from build123d import *

# Parameters (mm, degrees)
SKETCH_1_W                 = 44
SKETCH_1_H                 = 78
EXTRUDE_1_DEPTH            = 35
SHELL_1_T                  = -3
SHELL_1_THICKNESS_2_FACE_W = 75
SHELL_1_THICKNESS_2_FACE_H = 38
SHELL_1_THICKNESS_2_DEPTH  = 7
SKETCH_3_R                 = 3.6
CUT_EXTRUDE_1_DEPTH        = 4.1
CUT_EXTRUDE_2_REACH        = 53.284
SKETCH_4_R                 = 2.25
SKETCH_5_W                 = 3
SKETCH_5_H                 = 3
CUT_EXTRUDE_3_DEPTH        = 6
SKETCH_6_W                 = 8
SKETCH_6_H                 = 8
SKETCH_6_R                 = 1.75
EXTRUDE_2_DEPTH            = 8
CUT_EXTRUDE_4_DEPTH        = 2.6
CUT_EXTRUDE_5_REACH        = 90.034
SKETCH_8_R                 = 5


with BuildPart() as part:
    # 草圖1 → 填料-伸長1 (new body)
    with BuildSketch(Plane(origin=(0, 0, 0), x_dir=(1, 0, 0), z_dir=(0, 1, 0))):
        Rectangle(SKETCH_1_W, SKETCH_1_H)
    extrude(amount=EXTRUDE_1_DEPTH)

    # 薄殼1
    shell_1_openings = [part.faces().sort_by_distance(p)[0] for p in [
        (0, 17.5, 39),
    ]]
    offset(amount=SHELL_1_T, openings=shell_1_openings, kind=Kind.INTERSECTION)

    # 薄殼1 thickness 2 face (on inner face of the shell) → 薄殼1 thickness 2 (add)
    with BuildSketch(Plane(origin=(0, 3, 1.5), x_dir=(0, 0, -1), z_dir=(0, -1, 0))):
        Rectangle(SHELL_1_THICKNESS_2_FACE_W, SHELL_1_THICKNESS_2_FACE_H)
    extrude(amount=-SHELL_1_THICKNESS_2_DEPTH)

    # 草圖3 → 除料-伸長1 (cut)
    with BuildSketch(Plane(origin=(0, 10, 0), x_dir=(1, 0, 0), z_dir=(0, 1, 0))):
        with Locations(Location((0, 25, 0), (0, 0, 270))):
            Circle(SKETCH_3_R)
        with Locations(Location((0, -29, 0), (0, 0, 270))):
            Circle(SKETCH_3_R)
    extrude(amount=-CUT_EXTRUDE_1_DEPTH, mode=Mode.SUBTRACT)

    # 草圖4 → 除料-伸長2 (cut, up to next)
    with BuildSketch(Plane(origin=(0, 10, 0), x_dir=(1, 0, 0), z_dir=(0, 1, 0)), mode=Mode.PRIVATE) as cut_extrude_2_sk1:
        with Locations(Location((0, 25, 0), (0, 0, 270))):
            Circle(SKETCH_4_R)
    cut_extrude_2_tool1 = extrude(cut_extrude_2_sk1.sketch, amount=-CUT_EXTRUDE_2_REACH, mode=Mode.PRIVATE) & part.part
    # 草圖4 → 除料-伸長2 (cut, up to next)
    with BuildSketch(Plane(origin=(0, 10, 0), x_dir=(1, 0, 0), z_dir=(0, 1, 0)), mode=Mode.PRIVATE) as cut_extrude_2_sk2:
        with Locations(Location((0, -29, 0), (0, 0, 270))):
            Circle(SKETCH_4_R)
    cut_extrude_2_tool2 = extrude(cut_extrude_2_sk2.sketch, amount=-CUT_EXTRUDE_2_REACH, mode=Mode.PRIVATE) & part.part
    add(cut_extrude_2_tool1.solids().sort_by_distance((0, 10, -25))[0], mode=Mode.SUBTRACT)
    add(cut_extrude_2_tool2.solids().sort_by_distance((0, 10, 29))[0], mode=Mode.SUBTRACT)

    # 草圖5 → 除料-伸長3 (cut)
    with BuildSketch(Plane.XY.offset(39)):
        with Locations((20.5, 11.5)):
            Rectangle(SKETCH_5_W, SKETCH_5_H)
    extrude(amount=-CUT_EXTRUDE_3_DEPTH, mode=Mode.SUBTRACT)

    # 草圖6 → 填料-伸長2 (add)
    with BuildSketch(Plane.XY.offset(39)):
        with Locations((-26, 31)):
            Rectangle(SKETCH_6_W, SKETCH_6_H)
        with Locations((-26, 31)):
            Circle(SKETCH_6_R, mode=Mode.SUBTRACT)
        with Locations((-26, 4)):
            Rectangle(SKETCH_6_W, SKETCH_6_H)
        with Locations((-26, 4)):
            Circle(SKETCH_6_R, mode=Mode.SUBTRACT)
        with Locations((26, 4)):
            Rectangle(SKETCH_6_W, SKETCH_6_H)
        with Locations(Location((26, 4, 0), (0, 0, 180))):
            Circle(SKETCH_6_R, mode=Mode.SUBTRACT)
        with Locations((26, 31)):
            Rectangle(SKETCH_6_W, SKETCH_6_H)
        with Locations(Location((26, 31, 0), (0, 0, 180))):
            Circle(SKETCH_6_R, mode=Mode.SUBTRACT)
    extrude(amount=-EXTRUDE_2_DEPTH)

    # 草圖7 → 除料-伸長4 (cut)
    with BuildSketch(Plane(origin=(0, 0, 31), x_dir=(-1, 0, 0), z_dir=(0, 0, -1))):
        Polygon((27.58771324, 6.75), (29.175426481, 4), (27.58771324, 1.25), (24.41228676, 1.25), (22.824573519, 4), (24.41228676, 6.75), align=None)
        Polygon((-22.824573519, 31), (-24.41228676, 33.75), (-27.58771324, 33.75), (-29.175426481, 31), (-27.58771324, 28.25), (-24.41228676, 28.25), align=None)
        Polygon((-29.175426481, 4), (-27.58771324, 1.25), (-24.41228676, 1.25), (-22.824573519, 4), (-24.41228676, 6.75), (-27.58771324, 6.75), align=None)
        Polygon((24.41228676, 28.25), (22.824573519, 31), (24.41228676, 33.75), (27.58771324, 33.75), (29.175426481, 31), (27.58771324, 28.25), align=None)
    extrude(amount=-CUT_EXTRUDE_4_DEPTH, mode=Mode.SUBTRACT)

    # 草圖8 → 除料-伸長5 (cut, up to next)
    with BuildSketch(Plane.XY.offset(-36), mode=Mode.PRIVATE) as cut_extrude_5_sk1:
        with Locations((0, 20)):
            Circle(SKETCH_8_R)
    cut_extrude_5_tool1 = extrude(cut_extrude_5_sk1.sketch, amount=-CUT_EXTRUDE_5_REACH, mode=Mode.PRIVATE) & part.part
    add(cut_extrude_5_tool1.solids().sort_by_distance((0, 20, -36))[0], mode=Mode.SUBTRACT)


solid = part.part
Geometry: final body of the model. Coordinates: model frame, mm. A direction names the side the tool comes from. Give positions to 0.01 mm unless a question says otherwise; leave off trailing zeros. Write each loop counter-clockwise with the first axis right and the second up, starting at its lowest first coordinate (ties: lowest second). Pieces come first, ordered by that corner, then holes. Notation, with made-up numbers: (89, 30) -> (132, 30) arc R17 cw to (132, 41) -> close; hole circle Ø1 at (-22.75, 30.5). An arc over 180 degrees is marked (long way). Answer in a Markdown table with one row per item.
(1) Pin query (flat end, axial travel): pin 1 (6.5 mm diameter, centred on x = -4, y = 26.5, fed in from +Z); pin 2 (6 mm diameter, centred on y = 9.5, z = 23.5, fed in from -X); pin 3 (3 mm diameter, centred on y = 14, z = 23, fed in from +X). Return the tip coordinate at first contact, or that it passes through.
Answers below:
| item | result |
|---|---|
| pin 1 | z = -36 |
| pin 2 | x = -22 |
| pin 3 | x = 22 |
(2) Section query A-A on x = 26. Return loops of the section in (y, z).
Answers below:
| item | result |
|---|---|
| outline | (0, 31) -> (1.25, 31) -> (1.25, 33.6) -> (2.25, 33.6) -> (2.25, 39) -> (0, 39) -> close; (5.75, 33.6) -> (6.75, 33.6) -> (6.75, 31) -> (8, 31) -> (8, 39) -> (5.75, 39) -> close; (27, 31) -> (28.25, 31) -> (28.25, 33.6) -> (29.25, 33.6) -> (29.25, 39) -> (27, 39) -> close; (32.75, 33.6) -> (33.75, 33.6) -> (33.75, 31) -> (35, 31) -> (35, 39) -> (32.75, 39) -> close |
(3) Ray query, line 1 along Y through (x, z) = (-11, -17.5); line 2 along X through (y, z) = (2, -25); line 3 along X through (y, z) = (22, -25). Return the intervals inside material, ascending. Write a range as [from, to].
Answers below:
| item | result |
|---|---|
| line 1 | [0, 10], [32, 35] |
| line 2 | [-22, -2.25], [2.25, 22] |
| line 3 | [-22, -19], [19, 22] |
(4) Section query D-D on z = 14. Return loops of the section in (x, y), then the cut area to 3 significant figures.
Answers below:
| item | result |
|---|---|
| outline | (-22, 0) -> (22, 0) -> (22, 35) -> (-22, 35) -> close; hole (-19, 10) -> (19, 10) -> (19, 32) -> (-19, 32) -> close |
| area | 704 mm^2 |
(5) Draft query along Y for faces 5 (the flat face through (-23.63, 29.606, 32.282)), 6 (the flat face through (0, 0, -1)), 7 (the flat face through (0, 13, -39)). Return one class per face: +Y half, -Y half, draft (parallel to the pull), parting line (faces both ways), or undercut.
Answers below:
| item | result |
|---|---|
| face 5 | undercut |
| face 6 | -Y half |
| face 7 | draft |
(6) Set-up query: faces 1 (the flat face through (23.63, 2.606, 32.282)), 2 (the flat face through (26, 8, 35)), 3 (the flat face through (-26, 27, 35)), 4 (the flat face through (23, 32, 31)). Return all of +Z, -Z, +X, -X, +Y, -Y with unobstructed straight access to the full face (end or side cutting, diameter ignored); none if empty.
Answers below:
| item | result |
|---|---|
| face 1 | -Z |
| face 2 | +Z, -Z, +X |
| face 3 | +Z, -Z, -X |
| face 4 | -Z, +X, +Y, -Y |
(7) Section query B-B on y = 18.5. Return loops of the section in (x, z).
Answers below:
| item | result |
|---|---|
| outline | (-22, -39) -> (-4.77, -39) -> (-4.77, -36) -> (-19, -36) -> (-19, 39) -> (-22, 39) -> close; (4.77, -39) -> (22, -39) -> (22, 39) -> (19, 39) -> (19, -36) -> (4.77, -36) -> close |
(8) Section query C-C on z = 29. Return loops of the section in (x, y).
Answers below:
| item | result |
|---|---|
| outline | (-22, 0) -> (-2.25, 0) -> (-2.25, 5.9) -> (-3.6, 5.9) -> (-3.6, 10) -> (-19, 10) -> (-19, 32) -> (19, 32) -> (19, 10) -> (3.6, 10) -> (3.6, 5.9) -> (2.25, 5.9) -> (2.25, 0) -> (22, 0) -> (22, 35) -> (-22, 35) -> close |
